```python
from build123d import *

# Parameters (mm, degrees)
SKETCH1_R           = 4
SKETCH1_R_2         = 22.5
SKETCH1_R_3         = 1.5
BOSS_EXTRUDE1_DEPTH = 5


with BuildPart() as part:
    # Sketch1 → Boss-Extrude1 (new body)
    with BuildSketch(Plane.XY):
        with BuildLine():
            Line((-38.5, 32.5), (38.5, 32.5))
            ThreePointArc((38.5, 32.5), (71, 0), (38.5, -32.5))
            Line((38.5, -32.5), (-38.5, -32.5))
            ThreePointArc((-38.5, -32.5), (-71, 0), (-38.5, 32.5))
        make_face()
        with Locations((-38.5, 0)):
            Circle(SKETCH1_R, mode=Mode.SUBTRACT)
        with Locations((38.5, 0)):
            Circle(SKETCH1_R_2, mode=Mode.SUBTRACT)
        with Locations((-38.5, 22.5)):
            Circle(SKETCH1_R_3, mode=Mode.SUBTRACT)
        with Locations((-16, 0)):
            Circle(SKETCH1_R_3, mode=Mode.SUBTRACT)
        with Locations((-38.5, -22.5)):
            Circle(SKETCH1_R_3, mode=Mode.SUBTRACT)
        with Locations((-61, 0)):
            Circle(SKETCH1_R_3, mode=Mode.SUBTRACT)
        with Locations((11.5, 0)):
            Circle(SKETCH1_R_3, mode=Mode.SUBTRACT)
        with Locations((11.5, -25)):
            Circle(SKETCH1_R_3, mode=Mode.SUBTRACT)
        with Locations((11.5, 25)):
            Circle(SKETCH1_R_3, mode=Mode.SUBTRACT)
        with Locations((65.5, 0)):
            Circle(SKETCH1_R_3, mode=Mode.SUBTRACT)
        with Locations((-38.5, 8.5)):
            Circle(SKETCH1_R_3, mode=Mode.SUBTRACT)
        with Locations((-38.5, -8.5)):
            Circle(SKETCH1_R_3, mode=Mode.SUBTRACT)
        with Locations((38.5, 27)):
            Circle(SKETCH1_R_3, mode=Mode.SUBTRACT)
        with Locations((38.5, -27)):
            Circle(SKETCH1_R_3, mode=Mode.SUBTRACT)
        with BuildLine():
            Line((-2.25, 5), (-2.25, 15))
            ThreePointArc((-2.25, 15), (0, 17.25), (2.25, 15))
            Line((2.25, 15), (2.25, 5))
            ThreePointArc((2.25, 5), (0, 2.75), (-2.25, 5))
        make_face(mode=Mode.SUBTRACT)
    extrude(amount=BOSS_EXTRUDE1_DEPTH)


solid = part.part
```
Build history of the part. All positions in model axes, mm. A direction names the side the tool comes from. Coordinates: 2 decimals unless noted, no trailing zeros. Order: outer loops, then holes, each group sorted by start corner. A loop starts at its lowest first (then second) coordinate and runs counter-clockwise, first axis right, second up.
Item 1: Drop flat-ended pins along their axis: pin 1 Ø4 at (x, y) = (11.5, 25) entering from +Z; pin 2 Ø1.5 at (y, z) = (10, 3) entering from -X; pin 3 Ø2.5 at (y, z) = (12.5, 1.5) entering from +X; pin 4 Ø1.5 at (x, z) = (-51.5, 1.5) entering from +Y. Give the stop position or say it passes through.
Filled in:
pin 1: stops at z = 5
pin 2: stops at x = -69.66
pin 3: stops at x = 68.99
pin 4: stops at y = 30.1
Item 2: Saw through at C-C on z = 2.75. State how many separate pieces and enclosed holes the cut face has, then the cut area to 3 significant figures.
Filled in:
separate pieces: 1
enclosed holes: 15
area: 6,540 mm2
Item 3: Drill centre lines: L1, parallel to Y at x = -38.5, z = 2.3; L2, parallel to Y at x = 11.5, z = 4; L3, parallel to Y at x = 38.5, z = 2.5. Where is each one in solid material? Low to high.
Filled in:
L1: y = -32.5 to -24, -21 to -10, -7 to -4, 4 to 7, 10 to 21, 24 to 32.5
L2: y = -32.5 to -26.5, -23.5 to -1.5, 1.5 to 23.5, 26.5 to 32.5
L3: y = -32.5 to -28.5, -25.5 to -22.5, 22.5 to 25.5, 28.5 to 32.5
Item 4: Mould opens along X. For faces 1 (the flat face through (-1, 32.5, 2)), 2 (the cylindrical face through (70.992, 0.715, 2.465)), 3 (the flat face through (-2.25, 10, 2)) say: released by +X, released by -X, zero draft, split by the parting line, or undercut.
Filled in:
face 1: zero draft
face 2: released by +X
face 3: undercut
Item 5: Saw through at A-A on x = 0. List the corners of the cut face in (y, z).
Filled in:
outline: (-32.5, 0) - (2.75, 0) - (2.75, 5) - (-32.5, 5) - close; (17.25, 0) - (32.5, 0) - (32.5, 5) - (17.25, 5) - close
Item 6: Tool access for faces 4 (the flat face through (1, 0, 0)), 5 (the flat face through (2.25, 10, 2)): list every direction of +Z, -Z, +X, -X, +Y, -Y with a clear straight run to the whole face (end or side of a thin tool).
Filled in:
face 4: -Z, +X, -X, +Y, -Y
face 5: +Z, -Z
Item 7: Saw through at B-B on y = 11.5. List the corners of the cut face in (x, z).
Filled in:
outline: (-68.9, 0) - (-2.25, 0) - (-2.25, 5) - (-68.9, 5) - close; (2.25, 0) - (19.16, 0) - (19.16, 5) - (2.25, 5) - close; (57.84, 0) - (68.9, 0) - (68.9, 5) - (57.84, 5) - close
Item 8: Saw through at D-D on y = -8.5. List the corners of the cut face in (x, z).
Filled in:
outline: (-69.87, 0) - (-40, 0) - (-40, 5) - (-69.87, 5) - close; (-37, 0) - (17.67, 0) - (17.67, 5) - (-37, 5) - close; (59.33, 0) - (69.87, 0) - (69.87, 5) - (59.33, 5) - close
